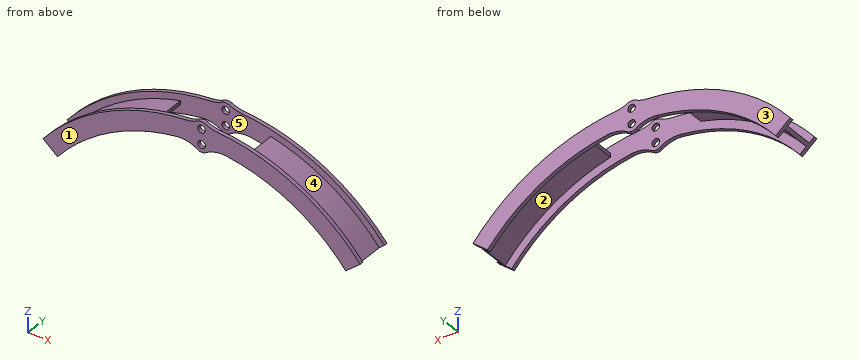
from build123d import *

# Parameters (mm, degrees)
SKETCH1_R           = 3.175
BOSS_EXTRUDE1_DEPTH = 3.175
BOSS_EXTRUDE2_DEPTH = 25.4
FILLET1_R           = 25.4
SKETCH4_W           = 38.1
SKETCH4_H           = 25.4
CUT_EXTRUDE1_DEPTH  = 254


# Read off the part's stored shape, not the designer's step: Boss-Extrude2
with BuildPart() as part:
    # Sketch1 → Boss-Extrude1 (new body)
    with BuildSketch(Plane(origin=(0, 0, 0), x_dir=(1, 0, 0), z_dir=(0, 1, 0))):
        with BuildLine():
            ThreePointArc((-133.675170743, 47.031446414), (-76.370132102, 1.839200867), (-5.549575239, -15.786213647))
            ThreePointArc((-5.549575239, -15.786213647), (0, -19.05), (5.549575239, -15.786213647))
            ThreePointArc((5.549575239, -15.786213647), (76.370132102, 1.839200867), (133.675170743, 47.031446414))
            Line((133.675170743, 47.031446414), (121.442816173, 57.15))
            ThreePointArc((121.442816173, 57.15), (69.968192782, 16.382290944), (6.348711382, 0.127921031))
            ThreePointArc((6.348711382, 0.127921031), (0, 6.35), (-6.348711382, 0.127921031))
            ThreePointArc((-6.348711382, 0.127921031), (-69.968192782, 16.382290944), (-121.442816173, 57.15))
            Line((-121.442816173, 57.15), (-133.675170743, 47.031446414))
        make_face()
        with Locations(Location((0, -12.7, 0), (0, 0, 270))):
            Circle(SKETCH1_R, mode=Mode.SUBTRACT)
        with Locations(Location((0, 0, 0), (0, 0, 270))):
            Circle(SKETCH1_R, mode=Mode.SUBTRACT)
    boss_extrude1 = extrude(amount=BOSS_EXTRUDE1_DEPTH)

    # Boss-Extrude2 outline → Boss-Extrude2 (add)
    with BuildSketch(Plane(origin=(0, 3.175, 0), x_dir=(1, 0, 0), z_dir=(0, 1, 0))):
        with BuildLine():
            ThreePointArc((2.08529156, -10.30580199), (72.444780746, 6.111748406), (129.393846644, 50.572940169))
            Line((129.393846644, 50.572940169), (126.947375729, 52.596650886))
            ThreePointArc((126.947375729, 52.596650886), (0, -7.14375), (-126.947375729, 52.596650886))
            Line((-126.947375729, 52.596650886), (-129.393846644, 50.572940169))
            ThreePointArc((-129.393846644, 50.572940169), (-72.444780746, 6.111748406), (-2.08529156, -10.30580199))
            ThreePointArc((-2.08529156, -10.30580199), (0, -9.525), (2.08529156, -10.30580199))
        make_face()
    extrude(amount=BOSS_EXTRUDE2_DEPTH)

    # Mirror1: Boss-Extrude1 across plane
    add(boss_extrude1.mirror(Plane(origin=(0, 15.875, 0), x_dir=(0, 0, 1), z_dir=(0, -1, 0))))

    # Fillet1
    fillet1_edges = [part.edges().sort_by_distance(p)[0] for p in [
        (-5.549575239, 1.5875, 15.786213647),
        (-6.348711382, 1.5875, -0.127921031),
        (6.348711382, 1.5875, -0.127921031),
        (5.549575239, 1.5875, 15.786213647),
        (5.549575239, 30.1625, 15.786213647),
        (-5.549575239, 30.1625, 15.786213647),
        (-6.348711382, 30.1625, -0.127921031),
        (6.348711382, 30.1625, -0.127921031),
    ]]
    fillet(fillet1_edges, radius=FILLET1_R)

    # Sketch4 → Cut-Extrude1 (cut)
    with BuildSketch(Plane.XY.offset(-52.596650886)):
        with Locations((-19.05, 15.875)):
            Rectangle(SKETCH4_W, SKETCH4_H)
        with Locations((19.05, 15.875)):
            Rectangle(SKETCH4_W, SKETCH4_H)
    extrude(amount=CUT_EXTRUDE1_DEPTH, mode=Mode.SUBTRACT)


solid = part.part
CAD build for the part. Positions are in the model's coordinates, mm. Face numbers are marked on the shaded views. A direction names the side the tool comes from. Round coordinates to 2 decimals unless told otherwise and drop trailing zeros. Loops run counter-clockwise (first coordinate to the right, second up) from the corner with the lowest first, then second, coordinate; pieces in that order, holes last.
(1) Cut at B-B (z = -22.5). Give the cut face in (x, y) (3 decimals).
(2) Cut at A-A (y = 13). Give the cut face in (x, z), plus the area to 3 significant figures.
(3) Drop flat-ended pins along their axis: pin 1 (4 mm diameter, centred on x = 0, z = 12.7, fed in from +Y); pin 2 (12 mm diameter, centred on y = 6, z = -14, fed in from -X); pin 3 (10 mm diameter, centred on x = 72.5, y = 11.5, fed in from +Z); pin 4 (1 mm diameter, centred on x = -54, y = 13.5, fed in from -Z). Give the stop position or say it passes through.
(4) Cut at D-D (z = 12.7). Give the cut face in (x, y) (3 decimals).
(5) Wall check: line 1 along Y through (x, z) = (-24.5, 10) (3 decimals); line 2 along X through (y, z) = (4, -23); line 3 along X through (y, z) = (14.5, -21). Give the ranges that are in metal, low to high.
(6) Cut at C-C (x = 33). Give the cut face in (y, z) (3 decimals).
(7) Two-plate mould, pull along Y, no slides. Class the marked faces 1, 2 and 3: +Y half, -Y half, draft (parallel to the pull), parting line (faces both ways), or undercut.
(8) Which spindle directions (+Z, -Z, +X, -X, +Y, -Y) get a long thin tool onto all of the face, cutting with end or side? Do the marked faces 4 and 5. Say none if no direction does.
Findings below:
1. outline: (-108.821, 0) - (-81.155, 0) - (-81.155, 3.175) - (-94.281, 3.175) - (-94.281, 28.575) - (-81.155, 28.575) - (-81.155, 31.75) - (-108.821, 31.75) - (-108.821, 28.575) - (-99.725, 28.575) - (-99.725, 3.175) - (-108.821, 3.175) - close; (81.155, 0) - (108.821, 0) - (108.821, 3.175) - (99.725, 3.175) - (99.725, 28.575) - (108.821, 28.575) - (108.821, 31.75) - (81.155, 31.75) - (81.155, 28.575) - (94.281, 28.575) - (94.281, 3.175) - (81.155, 3.175) - close
2. outline: (-129.39, -50.57) - (-126.95, -52.6) arc R164.75 cw to (-38.1, 2.68) - (-38.1, 5.94) arc R167.93 ccw to start; (38.1, 2.68) arc R164.75 cw to (126.95, -52.6) - (129.39, -50.57) arc R167.93 ccw to (38.1, 5.94) - close
2. area: 685 mm2
3. pin 1: passes through
3. pin 2: stops at x = -104.72
3. pin 3: stops at z = -3.84
3. pin 4: stops at z = -2.13
4. outline: (-33.038, 0) - (-3.175, 0) - (-3.175, 3.175) - (-33.038, 3.175) - close; (-33.038, 28.575) - (-3.175, 28.575) - (-3.175, 31.75) - (-33.038, 31.75) - close; (3.175, 0) - (33.038, 0) - (33.038, 3.175) - (3.175, 3.175) - close; (3.175, 28.575) - (33.038, 28.575) - (33.038, 31.75) - (3.175, 31.75) - close
5. line 1: y = 0 to 3.175, 28.575 to 31.75
5. line 2: x = -100.4 to -94.99, 94.99 to 100.4
5. line 3: x = -97.66 to -92.09, 92.09 to 97.66
6. outline: (0, -3.494) - (3.175, -3.494) - (3.175, 12.707) - (0, 12.707) - close; (28.575, -3.494) - (31.75, -3.494) - (31.75, 12.707) - (28.575, 12.707) - close
7. face 1: -Y half
7. face 2: undercut
7. face 3: +Y half
8. face 4: +Z, +X
8. face 5: none
